Check sheet for the modelled part. Datum: model origin and axes. Units: mm. A direction names the side the tool comes from. Give positions to 0.01 mm unless a question says otherwise; leave off trailing zeros. Write each loop counter-clockwise with the first axis right and the second up, starting at its lowest first coordinate (ties: lowest second). Pieces come first, ordered by that corner, then holes. Notation, with made-up numbers: M -38,78.25 L 20,78.25 A14 ccw 20,98.25 Z; hole C 53.25,56 d1. An arc over 180 degrees is marked long. One line per item, written item: value. Start each with the question number.
Autodesk Inventor part; units mm, degrees
ref_plane "YZ Plane" through (0, 0, 0) normal (1, 0, 0) x (0, 1, 0)
ref_plane "XZ Plane" through (0, 0, 0) normal (0, 1, 0) x (-1, 0, 0)
ref_plane "XY Plane" through (0, 0, 0) normal (0, 0, 1) x (1, 0, 0)
sketch "Sketch1" plane through (0, 0, 0) normal (0, 0, 1) x (1, 0, 0)
  line L0 (0, 0) -> (-7.5, 0)
  line L1 (-7.5, 0) -> (-7.5, 15)
  line L2 (-7.5, 15) -> (7.5, 15)
  line L3 (7.5, 15) -> (7.5, 0)
  line L4 (7.5, 0) -> (-7.5, 0)
  dimension "d55" = 7.5
  dimension "d56" = 15
  dimension "d57" = 15
extrude "Extrusion1" add sketch "Sketch1" along normal mid plane 15
sketch "Sketch11" plane through (0, 0, 7.5) normal (0, 0, 1) x (1, 0, 0)
  line L0 (7.5, 15) -> (-7.5, 15)
  line L1 (0, 15) -> (0, -25)
  line L2 (0, -25) -> (4.25, -25)
  line L3 (0, -25) -> (-4.25, -25)
  line L4 (-7.5, 0) -> (7.5, 0)
  line L5 (-4.25, -25) -> (-7.5, 0)
  line L6 (-7.5, 0) -> (7.5, 0)
  line L7 (7.5, 0) -> (4.25, -25)
  point P0 (0, 0)
  dimension "d58" = 40
  dimension "d59" = 4.25
  dimension "d60" = 4.25
extrude "Extrusion7" add sketch "Sketch11" against normal blind 15
sketch "Sketch13" plane through (0, 0, 0) normal (1, 0, 0) x (0, 1, 0)
  line L0 (15, -7.5) -> (15, 7.5)
  line L1 (15, 0) -> (-25, 0)
  line L2 (-25, 7.5) -> (-25, -7.5)
  line L3 (-25, 0) -> (-25, 4.25)
  line L4 (-25, 7.5) -> (-25, -7.5)
  line L5 (-25, 4.25) -> (-25, 0)
  line L6 (-25, 0) -> (-25, -4.25)
  line L7 (0, -7.5) -> (15, -7.5)
  line L8 (-25, -4.25) -> (0, -7.5)
  line L9 (0, -7.5) -> (0, 7.5)
  line L10 (0, 7.5) -> (-25, 4.25)
  line L11 (-25, 4.25) -> (-25, 7.5)
  line L12 (-25, 7.5) -> (0, 7.5)
  line L13 (-25, -4.25) -> (-25, -7.5)
  line L14 (-25, -7.5) -> (0, -7.5)
  line L15 (-25, -7.5) -> (0, -7.5)
  point P0 (0, 0)
  dimension "d68" = 40
  dimension "d69" = 4.25
  dimension "d70" = 4.25
extrude "Extrusion8" cut sketch "Sketch13" along normal through all both and the other way through all contours L14 L2 L8 | L10 L2 L12
sketch "Sketch15" plane through (-4.25, -25, -4.25) normal (0, -1, 0) x (1, 0, 0)
  line L0 (4.25, 4.25) -> (2.15, 4.25)
  line L1 (0, 8.5) -> (0, 0)
  line L2 (2.15, 4.25) -> (2.15, 2.15)
  line L3 (2.15, 2.15) -> (6.35, 2.15)
  line L4 (6.35, 2.15) -> (6.35, 6.35)
  line L5 (6.35, 6.35) -> (2.15, 6.35)
  line L6 (2.15, 6.35) -> (2.15, 4.25)
  point P0 (8.5, 8.5)
  point P1 (8.5, 0)
  dimension "d112" = 2.1
  dimension "d113" = 2.1
  dimension "d114" = 4.2
  dimension "d115" = 4.2
extrude "Extrusion9" cut sketch "Sketch15" against normal through all
sketch "Sketch16" plane through (0, 0, 7.5) normal (0, 0, 1) x (1, 0, 0)
  line L0 (0, 0) -> (4.9, 0)
  line L1 (-7.5, 0) -> (7.5, 0)
  line L2 (4.9, 0) -> (4.9, 16.5506)
  line L3 (0, 0) -> (-4.9, 0)
  line L4 (-4.9, 0) -> (-4.9, 16.5506)
  line L5 (-4.9, 16.5506) -> (4.9, 16.5506)
  dimension "d83" = 4.9
  dimension "d84" = 4.9
extrude "Extrusion10" cut sketch "Sketch16" against normal through all
sketch "Sketch17" plane through (7.5, 15, 7.5) normal (1, 0, 0) x (0, 0, -1)
  line L0 (15, 0) -> (0, 0)
  line L1 (0, 0) -> (7.5, 0)
  line L2 (7.5, 0) -> (7.5, -7.5)
  arc A0 (15, -7.5) -> (0, -7.5) centre (7.5, -7.5) ccw
  line L3 (0, 0) -> (0, -15)
  line L4 (0, -7.5) -> (0, 0)
  line L5 (0, 0) -> (15, 0)
  line L6 (15, -15) -> (15, 0)
  line L7 (15, 0) -> (15, -7.5)
  point P0 (7.5, -15)
  dimension "d87" = 7.5
extrude "Extrusion11" cut sketch "Sketch17" against normal through all
sketch "Sketch18" plane through (7.5, 0, 7.5) normal (1, 0, 0) x (0, 0, -1)
  line L0 (0, 0) -> (0, 15)
  line L1 (0, 15) -> (15, 15)
  line L2 (15, 15) -> (15, 0)
  line L3 (15, 0) -> (0, 0)
  line L4 (0, 15) -> (15, 0)
  line L5 (15, 15) -> (0, 0)
  circle A0 centre (7.5, 7.5) radius 4.15
  point P0 (7.5, 0)
  dimension "d90" = 15
  dimension "d91" = 8.3
extrude "Extrusion12" cut sketch "Sketch18" against normal blind 8.3 contours A0 L4 L5 | L5 L4 A0 | A0 L5 L4 | L4 L5 A0
sketch "Sketch19" plane through (-7.5, 0, -7.5) normal (-1, 0, 0) x (0, 0, 1)
  line L0 (0, 0) -> (0, 15)
  line L1 (0, 15) -> (15, 15)
  line L2 (15, 15) -> (15, 0)
  line L3 (15, 0) -> (0, 0)
  line L4 (15, 0) -> (0, 0)
  point P0 (7.5, 0)
  dimension "d94" = 15
extrude "Extrusion13" add sketch "Sketch19" along normal blind 3
sketch "Sketch20" plane through (-4.9, 0, 7.5) normal (1, 0, 0) x (0, 0, -1)
  line L0 (0, 0) -> (0, 15)
  line L1 (0, 0) -> (0, 15)
  line L2 (0, 15) -> (15, 15)
  line L3 (15, 0) -> (0, 0)
  line L4 (15, 15) -> (15, 0)
  line L5 (15, 0) -> (0, 0)
  line L6 (0, 0) -> (15, 15)
  line L7 (0, 15) -> (15, 0)
  circle A0 centre (7.5, 7.5) radius 4.15
  point P0 (7.5, 0)
  dimension "d97" = 15
  dimension "d98" = 8.3
extrude "Extrusion14" cut sketch "Sketch20" against normal blind 2.6 contours A0 L7 L6 | L6 L7 A0 | A0 L6 L7 | L7 L6 A0
sketch "Sketch21" plane through (-10.5, 0, -7.5) normal (-1, 0, 0) x (0, 0, 1)
  line L0 (0, 7.5) -> (0, 0)
  line L1 (15, 0) -> (15, 15)
  line L2 (0, 0) -> (15, 15)
  line L3 (0, 15) -> (0, 0)
  line L4 (15, 15) -> (0, 15)
  line L5 (0, 15) -> (15, 0)
  line L6 (7.5, 7.5) -> (7.5, 10.5)
  line L7 (7.5, 10.5) -> (10.5, 10.5)
  line L8 (10.5, 10.5) -> (10.5, 4.5)
  line L9 (10.5, 4.5) -> (4.5, 4.5)
  line L10 (4.5, 4.5) -> (4.5, 10.5)
  line L11 (4.5, 10.5) -> (10.5, 10.5)
  point P0 (7.5, 0)
  dimension "d101" = 3
  dimension "d102" = 3
  dimension "d103" = 6
  dimension "d104" = 6
extrude "Extrusion15" cut sketch "Sketch21" against normal blind 3 contours L10 L5 L2 | L2 L5 L9 | L11 L6 L5 | L6 L7 L2 | L2 L8 L5
sketch "Sketch23" plane through (-4.9, 0, 7.5) normal (1, 0, 0) x (0, 0, -1)
  line L0 (0, 0) -> (0, 15)
  line L1 (0, 0) -> (0, 15)
  line L2 (0, 15) -> (15, 15)
  line L3 (15, 15) -> (15, 0)
  line L4 (15, 0) -> (0, 0)
  line L5 (0, 15) -> (7.5, 15)
  arc A0 (15, 7.5) -> (0, 7.5) centre (7.5, 7.5) ccw
  line L6 (0, 7.5) -> (0, 15)
  line L7 (15, 15) -> (15, 7.5)
  point P0 (7.5, 0)
  point P1 (0, 7.5)
  dimension "d107" = 15
extrude "Extrusion16" cut sketch "Sketch23" against normal through all contours L0 L2 A0 | L2 L3 A0
fillet "Fillet2" radius 5 1 edges at (-7.5, 0, 0)
sketch "Sketch25" plane through (-10.5, 0, -7.5) normal (-1, 0, 0) x (0, 0, 1)
  point P0 (7.5, 0)
equation "\"d92\" = d91"
equation "\"d105\" = d101"
properties part number "Hip Joint 2"
1) Material ranges on L1, parallel to Z at x = 5.6, y = 7.5; L2, parallel to X at y = 2, z = -5.75; L3, parallel to Z at x = 1.25, y = -8, recorded low to high. Write a range as from..to.
2) Cross-section at C-C (x = 1). Record the boundary of the cut face in (y, z).
3) Cross-section at D-D (x = -8.25). Record the boundary of the cut face in (y, z), plus the area to 3 significant figures.
4) Gauge pin test, flat ends, axial feed: pin 1 (1 mm diameter, centred on y = -7, z = -2.5, fed in from +X) (3 decimals); pin 2 (0.9 mm diameter, centred on y = 11, z = -1, fed in from +X); pin 3 (8 mm diameter, centred on y = -20, z = -3.5, fed in from -X). Record the tip position at first contact, or that the pin passes through.
5) Cross-section at A-A (y = -6). Record the boundary of the cut face in (x, z).
6) Tool access check on faces 4 (the cylindrical face through (-6.182, 11.615, 0.54)), 5 (the cylindrical face through (-8, 15, 0)), 6 (the flat face through (0, -13, 2.1)), 7 (the flat face through (4.9, 4, -3)), 8 (the flat face through (5.9, -12.3, 0.1)). Record the directions out of +Z, -Z, +X, -X, +Y, -Y that give a thin tool (end or side, any length) a straight path to the whole face; none if there is none.
7) Draft check along X on faces 1 (the flat face through (7.5, 4, 3)), 2 (the flat face through (0, -13, -2.1)), 3 (the flat face through (-8, 4, -7.5)). Enter one of: released by +X, released by -X, zero draft, split by the parting line, or undercut.
8) Cross-section at B-B (z = 0). Record the boundary of the cut face in (x, y), plus the area to 3 significant figures.
Data:
1. L1: z = -7.5..-4.15, 4.15..7.5
1. L2: x = -10.5..-4.9, 4.9..7.5
1. L3: z = -6.46..-2.1, 2.1..6.46
2. outline: M -25,-4.25 L 0,-7.5 L 0,-2.1 L -25,-2.1 Z; M -25,2.1 L 0,2.1 L 0,7.5 L -25,4.25 Z
3. outline: M -1.4,-7.32 L 0,-7.5 L 7.5,-7.5 A7.5 ccw 7.5,7.5 L 0,7.5 L -1.4,7.32 Z; hole M 4.5,-3 L 10.5,-3 L 10.5,3 L 4.5,3 Z
3. area: 186 mm2
4. pin 1: stops at x = 6.655
4. pin 2: stops at x = -7.5
4. pin 3: stops at x = -5.42
5. outline: M -6.72,-6.72 L 6.72,-6.72 L 6.72,6.72 L -6.72,6.72 Z; hole M -2.1,-2.1 L 2.1,-2.1 L 2.1,2.1 L -2.1,2.1 Z
6. face 4: +X
6. face 5: +X, -X, +Y
6. face 6: +Y, -Y
6. face 7: +Z, -Z, +Y
6. face 8: +Z, -Z, +X, -Y
7. face 1: released by +X
7. face 2: undercut
7. face 3: zero draft
8. outline: M -10.5,0 A5 cw -6.96,-4.15 L -4.25,-25 L -2.1,-25 L -2.1,0 L -4.9,0 L -4.9,3.35 L -7.5,3.35 L -7.5,4.5 L -10.5,4.5 Z; M -10.5,10.5 L -7.5,10.5 L -7.5,11.65 L -4.9,11.65 L -4.9,15 L -10.5,15 Z; M 2.1,-25 L 4.25,-25 L 7.5,0 L 7.5,3.35 L 4.9,3.35 L 4.9,0 L 2.1,0 Z; M 4.9,11.65 L 7.5,11.65 L 7.5,15 L 4.9,15 Z
8. area: 254 mm2
